Could you check a few things on this model? Use its own coordinates, in mm. A direction names the side the tool comes from. Round coordinates to 2 decimals unless told otherwise and drop trailing zeros. Loops run counter-clockwise (first coordinate to the right, second up) from the corner with the lowest first, then second, coordinate; pieces in that order, holes last. Notation, with made-up numbers: M -12.75,-8.75 L 31.25,-8.75 A19 cw 31.25,16.25 Z; hole C 16.5,39 d1. An arc over 180 degrees is marked long. Answer in a Markdown table with one row per item.
```python
from build123d import *

# Parameters (mm, degrees)
ESQUISSE1_R        = 1.5
BOSS_EXTRU_1_DEPTH = 2.4
ESQUISSE2_W        = 9
ESQUISSE2_H        = 4.4
BOSS_EXTRU_2_DEPTH = 9


with BuildPart() as part:
    # Esquisse1 → Boss.-Extru.1 (new body)
    with BuildSketch(Plane.XY):
        Polygon((0, 30), (0, 3), (3, 0), (30, 0), (33, 3), (33, 30), (30, 33), (3, 33), align=None)
        with Locations((4.5, 28.5)):
            Circle(ESQUISSE1_R, mode=Mode.SUBTRACT)
        with Locations(Location((28.5, 28.5, 0), (0, 0, 180))):
            Circle(ESQUISSE1_R, mode=Mode.SUBTRACT)
        with Locations(Location((4.5, 4.5, 0), (0, 0, 180))):
            Circle(ESQUISSE1_R, mode=Mode.SUBTRACT)
        with Locations((28.5, 4.5)):
            Circle(ESQUISSE1_R, mode=Mode.SUBTRACT)
    extrude(amount=BOSS_EXTRU_1_DEPTH)

    # Esquisse2 → Boss.-Extru.2 (add)
    with BuildSketch(Plane.XY.offset(2.4)):
        with Locations((16.5, 16.5)):
            Rectangle(ESQUISSE2_W, ESQUISSE2_H)
    extrude(amount=BOSS_EXTRU_2_DEPTH)


solid = part.part
```
1) Will these pins go through, and if not, where does the flat tip stop? P1, Ø6, axis at x = 21.5, z = 7.5, coming from the +Y side; P2, Ø4, axis at x = 4.5, y = 4.5, coming from the +Z side; P3, Ø3, axis at x = 21.5, z = 8.5, coming from the -Y side; P4, Ø2.5, axis at x = 4.5, y = 28.5, coming from the -Z side.
Computed:
| item | result |
|---|---|
| P1 | stops at y = 18.7 |
| P2 | stops at z = 2.4 |
| P3 | stops at y = 14.3 |
| P4 | passes through |
2) I want a section at B-B, the plane x = 4.5. Please give me the cut outline in (y, z), plus the area to 3 significant figures.
Computed:
| item | result |
|---|---|
| outline | M 0,0 L 3,0 L 3,2.4 L 0,2.4 Z; M 6,0 L 27,0 L 27,2.4 L 6,2.4 Z; M 30,0 L 33,0 L 33,2.4 L 30,2.4 Z |
| area | 64.8 mm² |
3) Which directions (+Z, -Z, +X, -X, +Y, -Y) give clear straight access to the entire face, cutting with the end or side of a thin tool? Please do faces 1 (the face through (12, 16, 7)), 2 (the face through (21, 16, 7)), 3 (the face through (16, 18.7, 7)), 4 (the face through (16, 14.3, 7)).
Computed:
| item | result |
|---|---|
| face 1 | +Z, -X, +Y, -Y |
| face 2 | +Z, +X, +Y, -Y |
| face 3 | +Z, +X, -X, +Y |
| face 4 | +Z, +X, -X, -Y |
4) I want a section at D-D, the plane x = 19. Please give me the cut outline in (y, z).
Computed:
| item | result |
|---|---|
| outline | M 0,0 L 33,0 L 33,2.4 L 18.7,2.4 L 18.7,11.4 L 14.3,11.4 L 14.3,2.4 L 0,2.4 Z |
5) If we mould it in two halves opening along Y, with no side actions, what happens to faces 5 (the face through (29.61, 27.49, 1.18)), 6 (the face through (16, 17, 0)), 7 (the face through (16, 0, 1))? For each: released by +Y, released by -Y, zero draft, split by the parting line, or undercut.
Computed:
| item | result |
|---|---|
| face 5 | undercut |
| face 6 | zero draft |
| face 7 | released by -Y |
6) I want a section at A-A, the plane z = 1.25. Please give me the cut outline in (x, y), plus the area to 3 significant figures.
Computed:
| item | result |
|---|---|
| outline | M 0,3 L 3,0 L 30,0 L 33,3 L 33,30 L 30,33 L 3,33 L 0,30 Z; hole C 4.5,4.5 d3; hole C 4.5,28.5 d3; hole C 28.5,4.5 d3; hole C 28.5,28.5 d3 |
| area | 1,040 mm² |
7) I need wall thicknesses on line 1 (Y direction, x = 28.5, z = 1.2); line 2 (Z direction, x = 17, y = 13); line 3 (Y direction, x = 14, z = 3). Which ranges of each line are inside material? Lowest first, please.
Computed:
| item | result |
|---|---|
| line 1 | y = 0 to 3, 6 to 27, 30 to 33 |
| line 2 | z = 0 to 2.4 |
| line 3 | y = 14.3 to 18.7 |
